The figure shows three views and two pictorial views of one solid part (mm, origin at its lowest corner). Answer the questions. A direction names the side the tool comes from. Coordinates: 2 decimals unless noted, no trailing zeros. Order: outer loops, then holes, each group sorted by start corner. A loop starts at its lowest first (then second) coordinate and runs counter-clockwise, first axis right, second up. Notation, with made-up numbers: (8, -0.75) -> (41, -0.75) arc R16 ccw to (41, 26.25) -> close; hole circle Ø5 at (69.5, -3). An arc over 180 degrees is marked (long way). Return JSON: item names as keys, results as strings. Group by question number.
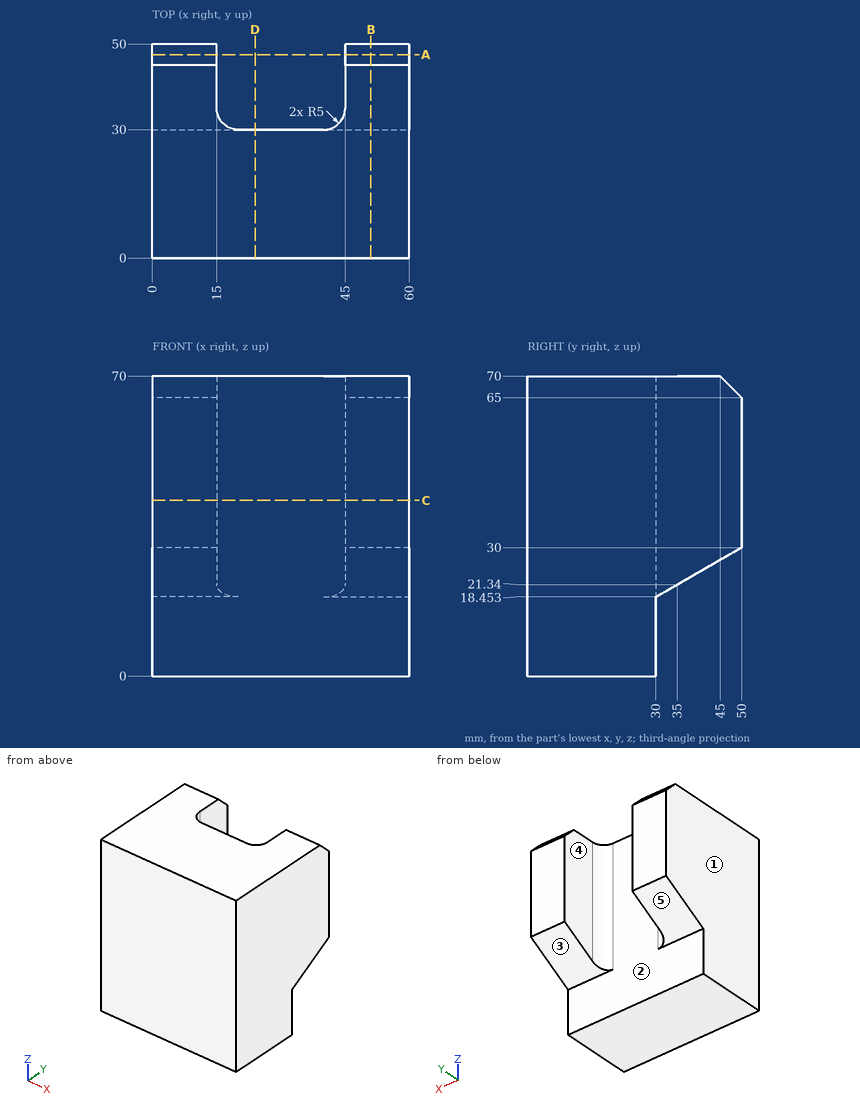
1. Given pin 1 (10 mm diameter, centred on x = 30, z = 30.5, fed in from +Y); pin 2 (8 mm diameter, centred on x = 10.5, y = 43, fed in from -Z), each flat-ended and moving along its own axis, determine where each tip first touches the part or whether it passes through.
2. Find section A-A on y = 47.5. Determine the outline of the cut face in (x, z).
3. For a pull along X with two mould halves and no side action, classify the marked faces 1, 2 and 3 as released by +X, released by -X, zero draft, split by the parting line, or undercut.
4. Find section C-C on z = 41. Determine the outline of the cut face in (x, y).
5. Find section D-D on x = 24. Determine the outline of the cut face in (y, z).
6. Straight lines are drawn through the part: L1, parallel to Y at x = 10, z = 7.5; L2, parallel to X at y = 36.5, z = 58.5; L3, parallel to X at y = 33.5, z = 48. For each, find the intervals that lie inside material, in ascending order.
7. Which of the six approach directions +Z, -Z, +X, -X, +Y, -Y give full straight-line access (tool end or side, diameter ignored) to the marked faces 4 and 5?
8. Find section B-B on x = 51. Determine the outline of the cut face in (y, z), and give its area (3 significant figures).
Result:
{
 "1": {"pin 1": "y = 30", "pin 2": "z = 23.65"},
 "2": {"outline": "(0, 28.56) -> (15, 28.56) -> (15, 67.5) -> (0, 67.5) -> close; (45, 28.56) -> (60, 28.56) -> (60, 67.5) -> (45, 67.5) -> close"},
 "3": {"face 1": "released by -X", "face 2": "undercut", "face 3": "zero draft"},
 "4": {"outline": "(0, 0) -> (60, 0) -> (60, 50) -> (45, 50) -> (45, 35) arc R5 cw to (40, 30) -> (20, 30) arc R5 cw to (15, 35) -> (15, 50) -> (0, 50) -> close"},
 "5": {"outline": "(0, 0) -> (30, 0) -> (30, 70) -> (0, 70) -> close"},
 "6": {"L1": "0 to 30", "L2": "0 to 15, 45 to 60", "L3": "0 to 15.23, 44.77 to 60"},
 "7": {"face 4": "+Z, -Z, +Y", "face 5": "-Z, +X, -X, +Y"},
 "8": {"outline": "(0, 0) -> (30, 0) -> (30, 18.45) -> (50, 30) -> (50, 65) -> (45, 70) -> (0, 70) -> close", "area": "3,000 mm^2"}
}
